Could you check a few things on this drawing? It's one solid part, dimensions in mm from its lowest x, y, z. Round coordinates to 2 decimals unless told otherwise and drop trailing zeros. Order: outer loops, then holes, each group sorted by start corner. A loop starts at its lowest first (then second) coordinate and runs counter-clockwise, first axis right, second up. Notation, with made-up numbers: M 55,-25 L 110,-25 A21 ccw 110,-10 Z; hole C -0.5,16 d1. An arc over 180 degrees is marked long. Answer as CSV lines item,"result". Start each with the question number.
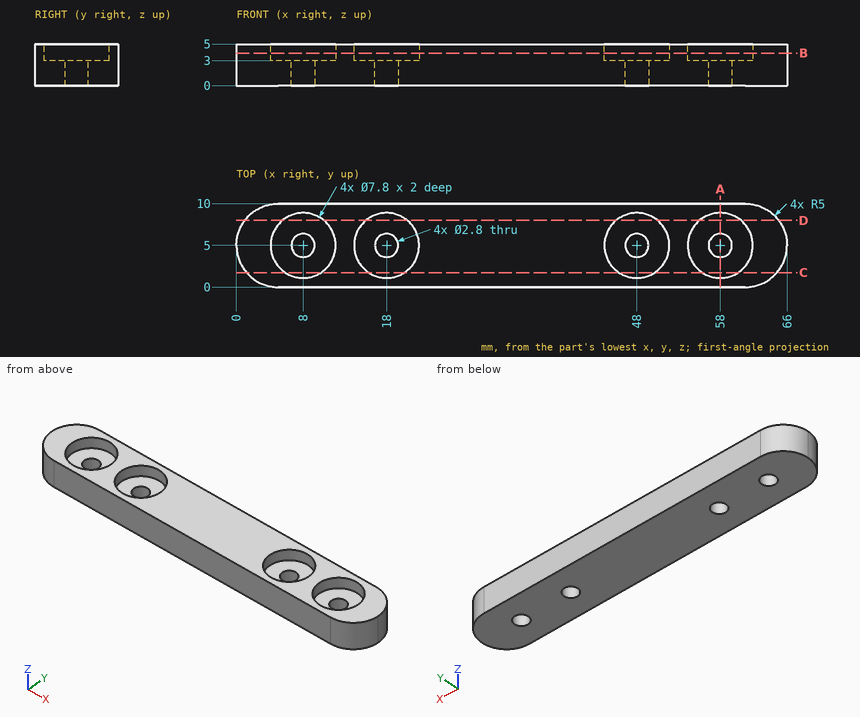
Item 1: If we section it at C-C on y = 1.75: Please give me the cut outline in (x, z), and give its area (4 significant figures).
Item 2: If we section it at A-A on x = 58: Please give me the cut outline in (y, z), and give its area (3 significant figures).
Item 3: If we section it at D-D on y = 8: Please give me the cut outline in (x, z), and give its area (3 significant figures).
Item 4: For P1, Ø3.5, axis at x = 18, y = 5, coming from the +Z side; P2, Ø1.5, axis at y = 6, z = 1, coming from the +X side; P3, Ø1, axis at y = 8, z = 2.5, coming from the +X side, each with a flat end and sliding along its axis, tell me the tip position at first contact or that it passes through.
Item 5: If I drill on line 1 along Y through (x, z) = (58, 0.7); line 2 along X through (y, z) = (8, 4.85); line 3 along Y through (x, z) = (8, 3.9), over which ranges is the centre line in solid material (lowest first)?
Item 6: If we section it at B-B on z = 3.9: Count the separate pieces of the cut face and the enclosed holes in it, and give its area (3 significant figures).
Geometry says:
1,outline,"M 1.2,0 L 64.8,0 L 64.8,5 L 60.16,5 L 60.16,3 L 55.84,3 L 55.84,5 L 50.16,5 L 50.16,3 L 45.84,3 L 45.84,5 L 20.16,5 L 20.16,3 L 15.84,3 L 15.84,5 L 10.16,5 L 10.16,3 L 5.84,3 L 5.84,5 L 1.2,5 Z"
1,area,"283.5 mm²"
2,outline,"M 0,0 L 3.6,0 L 3.6,3 L 1.1,3 L 1.1,5 L 0,5 Z; M 6.4,0 L 10,0 L 10,5 L 8.9,5 L 8.9,3 L 6.4,3 Z"
2,area,"26.0 mm²"
3,outline,"M 1,0 L 65,0 L 65,5 L 60.49,5 L 60.49,3 L 55.51,3 L 55.51,5 L 50.49,5 L 50.49,3 L 45.51,3 L 45.51,5 L 20.49,5 L 20.49,3 L 15.51,3 L 15.51,5 L 10.49,5 L 10.49,3 L 5.51,3 L 5.51,5 L 1,5 Z"
3,area,"280 mm²"
4,P1,"z = 3"
4,P2,"x = 65.99"
4,P3,"x = 65.33"
5,line 1,"0 to 3.6, 6.4 to 10"
5,line 2,"1 to 5.51, 10.49 to 15.51, 20.49 to 45.51, 50.49 to 55.51, 60.49 to 65"
5,line 3,"0 to 1.1, 8.9 to 10"
6,separate pieces,"1"
6,enclosed holes,"4"
6,area,"447 mm²"
